The listing builds one solid part. Answer for the finished solid, in the listing's coordinates (mm). A direction names the side the tool comes from. Coordinates: 2 decimals unless noted, no trailing zeros. Order: outer loops, then holes, each group sorted by start corner. A loop starts at its lowest first (then second) coordinate and runs counter-clockwise, first axis right, second up. Notation, with made-up numbers: (30.5, -26.5) -> (41.5, -26.5) arc R24 ccw to (41.5, -12.5) -> close; hole circle Ø9 at (71.5, 5). An arc over 180 degrees is marked (long way). Write item = value, one per line.
from build123d import *

# Parameters (mm, degrees)
F0_W     = 228.6
F0_H     = 177.8
F1_DEPTH = 12.7
F3_D     = 5.1054
F5_DEPTH = 12.701


with BuildPart() as f1:
    # F0 (on Top) → F1 (new body)
    with BuildSketch(Plane.XY):
        with Locations((-114.3, 88.9)):
            Rectangle(F0_W, F0_H)
    extrude(amount=F1_DEPTH)

    # F3 (through all)
    with Locations(Plane.XY.offset(12.7)):
        with Locations((-12.7, 38.1), (-12.7, 165.1), (-215.9, 38.1), (-215.9, 165.1)):
            Hole(F3_D / 2)

    # F4 (on face) → F5 (cut, through all)
    with BuildSketch(Plane.XY.offset(12.7)):
        with BuildLine():
            ThreePointArc((-24.60625, 120.65), (-21.43125, 117.475), (-18.25625, 120.65))
            Line((-18.25625, 120.65), (-18.25625, 146.05))
            ThreePointArc((-18.25625, 146.05), (-21.43125, 149.225), (-24.60625, 146.05))
            Line((-24.60625, 146.05), (-24.60625, 120.65))
        make_face()
        with BuildLine():
            ThreePointArc((-18.25625, 82.55), (-21.43125, 85.725), (-24.60625, 82.55))
            Line((-24.60625, 82.55), (-24.60625, 57.15))
            ThreePointArc((-24.60625, 57.15), (-21.43125, 53.975), (-18.25625, 57.15))
            Line((-18.25625, 57.15), (-18.25625, 82.55))
        make_face()
        with BuildLine():
            Line((-203.99375, 120.65), (-203.99375, 146.05))
            ThreePointArc((-203.99375, 146.05), (-207.16875, 149.225), (-210.34375, 146.05))
            Line((-210.34375, 146.05), (-210.34375, 120.65))
            ThreePointArc((-210.34375, 120.65), (-207.16875, 117.475), (-203.99375, 120.65))
        make_face()
        with BuildLine():
            ThreePointArc((-210.34375, 57.15), (-207.16875, 53.975), (-203.99375, 57.15))
            Line((-203.99375, 57.15), (-203.99375, 82.55))
            ThreePointArc((-203.99375, 82.55), (-207.16875, 85.725), (-210.34375, 82.55))
            Line((-210.34375, 82.55), (-210.34375, 57.15))
        make_face()
    extrude(amount=-F5_DEPTH, mode=Mode.SUBTRACT)


solid = f1.part
Q1. The mould has two halves that part along Y. Classify faces 1 (the face through (-116, 0, 6)), 2 (the face through (-116, 90, 12.7)), 3 (the face through (-207.239, 53.976, 6.439)): released by +Y, released by -Y, zero draft, split by the parting line, or undercut.
The answers:
face_1 = released by -Y
face_2 = zero draft
face_3 = undercut
Q2. Section A-A, the plane x = -12.7 is taken. Give the vertices of the cut face in (y, z), plus the area to 3 significant figures.
The answers:
outline = (0, 0) -> (35.55, 0) -> (35.55, 12.7) -> (0, 12.7) -> close; (40.65, 0) -> (162.55, 0) -> (162.55, 12.7) -> (40.65, 12.7) -> close; (167.65, 0) -> (177.8, 0) -> (177.8, 12.7) -> (167.65, 12.7) -> close
area = 2,130 mm2
Q3. A tool of negligible diameter and unlimited length cuts with its end or side. For faces 4 (the face through (-18.256, 70, 6)), 5 (the face through (0, 88, 6)), from which of +Z, -Z, +X, -X, +Y, -Y can it reach the whole face along a straight path? Write none if from no direction.
The answers:
face_4 = +Z, -Z
face_5 = +Z, -Z, +X, +Y, -Y
Q4. Find the intervals of material crossed by line 1 along X through (y, z) = (143, 11.25); line 2 along Y through (x, z) = (-12.7, 4); line 3 along X through (y, z) = (165.1, 8.5), in increasing order.
The answers:
line_1 = -228.6 to -210.34, -203.99 to -24.61, -18.26 to 0
line_2 = 0 to 35.55, 40.65 to 162.55, 167.65 to 177.8
line_3 = -228.6 to -218.45, -213.35 to -15.25, -10.15 to 0
Q5. Section B-B, the plane y = 165.1 is taken. Give the vertices of the cut face in (x, z).
The answers:
outline = (-228.6, 0) -> (-218.45, 0) -> (-218.45, 12.7) -> (-228.6, 12.7) -> close; (-213.35, 0) -> (-15.25, 0) -> (-15.25, 12.7) -> (-213.35, 12.7) -> close; (-10.15, 0) -> (0, 0) -> (0, 12.7) -> (-10.15, 12.7) -> close
Q6. Section C-C, the plane z = 3.5 is taken. Give the number of separate pieces and of enclosed holes in the cut face, plus the area to 3 significant figures.
The answers:
separate_pieces = 1
enclosed_holes = 8
area = 39,800 mm2
